```python
from build123d import *

# Parameters (mm, degrees)
BOSS_EXTRUDE1_DEPTH = 20
SKETCH2_R           = 5
BOSS_EXTRUDE2_DEPTH = 10
SKETCH3_R           = 11.25
CUT_EXTRUDE1_DEPTH  = 10
FILLET1_R           = 2.5
FILLET2_R           = 2.5


with BuildPart() as part:
    # Sketch1 → Boss-Extrude1 (new body)
    with BuildSketch(Plane.XY):
        with BuildLine():
            Line((-49.078947743, 24.658688111), (-53.195876289, 25))
            ThreePointArc((-53.195876289, 25), (-78.174127632, -1.04257365), (-51.112542955, -24.913043215))
            Line((-51.112542955, -24.913043215), (68.054123711, -14.947825929))
            ThreePointArc((68.054123711, -14.947825929), (81.804122753, 0.005360617), (68.04343945, 14.948715547))
            Line((68.04343945, 14.948715547), (-49.078947743, 24.658688111))
        make_face()
    extrude(amount=BOSS_EXTRUDE1_DEPTH)

    # Sketch2 → Boss-Extrude2 (add)
    with BuildSketch(Plane(origin=(0, 0, 0), x_dir=(-1, 0, 0), z_dir=(0, 0, -1))):
        with Locations(Location((-66.804123711, 0, 0), (0, 0, 180))):
            Circle(SKETCH2_R)
    extrude(amount=BOSS_EXTRUDE2_DEPTH)

    # Sketch3 → Cut-Extrude1 (cut)
    with BuildSketch(Plane.XY.offset(20)):
        with Locations((-53.195876289, 0)):
            Circle(SKETCH3_R)
    extrude(amount=-CUT_EXTRUDE1_DEPTH, mode=Mode.SUBTRACT)

    # Fillet1
    # the kernel refuses this fillet: 2.5 mm, written as the material it takes off along each edge
    with BuildSketch(Plane(origin=(66.804123711, 0, 20), x_dir=(0.08333333333333336, -0.9965217285917832, 0), z_dir=(-0.9965217285917832, -0.08333333333333336, 0))) as fillet1_piece_1:
        with BuildLine():
            CenterArc((15 - FILLET1_R, -FILLET1_R), FILLET1_R, 0, 90)
            Line((15 - FILLET1_R, 0), (15 - FILLET1_R, FILLET1_R * 0.02))
            Line((15 - FILLET1_R, FILLET1_R * 0.02), (15 + FILLET1_R * 0.02, FILLET1_R * 0.02))
            Line((15 + FILLET1_R * 0.02, FILLET1_R * 0.02), (15 + FILLET1_R * 0.02, -FILLET1_R))
            Line((15 + FILLET1_R * 0.02, -FILLET1_R), (15, -FILLET1_R))
        make_face()
    revolve(axis=Axis((66.804123711, 0, 20), (0, 0, 1)), revolution_arc=170.480568403, mode=Mode.SUBTRACT)
    with BuildSketch(Plane(origin=(-55.68732888, 25.206552623, 20), x_dir=(-0.08262104926117214, -0.9965810364536258, 0), z_dir=(0.9965810364536258, -0.08262104926117214, 0))) as fillet1_piece_2:
        with BuildLine():
            CenterArc((FILLET1_R, FILLET1_R), FILLET1_R, 180, 90)
            Line((0, FILLET1_R), (-FILLET1_R * 0.02, FILLET1_R))
            Line((-FILLET1_R * 0.02, FILLET1_R), (-FILLET1_R * 0.02, -FILLET1_R * 0.02))
            Line((-FILLET1_R * 0.02, -FILLET1_R * 0.02), (FILLET1_R, -FILLET1_R * 0.02))
            Line((FILLET1_R, -FILLET1_R * 0.02), (FILLET1_R, 0))
        make_face()
    extrude(amount=124.155250606, mode=Mode.SUBTRACT)
    with BuildSketch(Plane(origin=(-53.195876289, 0, 20), x_dir=(0.10000205270336067, 0.994987230800031, 0), z_dir=(0.994987230800031, -0.10000205270336067, 0))) as fillet1_piece_3:
        with BuildLine():
            CenterArc((25 - FILLET1_R, -FILLET1_R), FILLET1_R, 0, 90)
            Line((25 - FILLET1_R, 0), (25 - FILLET1_R, FILLET1_R * 0.02))
            Line((25 - FILLET1_R, FILLET1_R * 0.02), (25 + FILLET1_R * 0.02, FILLET1_R * 0.02))
            Line((25 + FILLET1_R * 0.02, FILLET1_R * 0.02), (25 + FILLET1_R * 0.02, -FILLET1_R))
            Line((25 + FILLET1_R * 0.02, -FILLET1_R), (25, -FILLET1_R))
        make_face()
    revolve(axis=Axis((-53.195876289, 0, 20), (0, 0, 1)), revolution_arc=190.519480528, mode=Mode.SUBTRACT)
    with BuildSketch(Plane(origin=(-51.112542955, -24.913043215, 20), x_dir=(0, 0, -1), z_dir=(0.9965217285917832, 0.08333333333333336, 0))) as fillet1_piece_4:
        with BuildLine():
            CenterArc((FILLET1_R, FILLET1_R), FILLET1_R, 180, 90)
            Line((0, FILLET1_R), (-FILLET1_R * 0.02, FILLET1_R))
            Line((-FILLET1_R * 0.02, FILLET1_R), (-FILLET1_R * 0.02, -FILLET1_R * 0.02))
            Line((-FILLET1_R * 0.02, -FILLET1_R * 0.02), (FILLET1_R, -FILLET1_R * 0.02))
            Line((FILLET1_R, -FILLET1_R * 0.02), (FILLET1_R, 0))
        make_face()
    extrude(amount=119.582607431, mode=Mode.SUBTRACT)

    # Fillet2
    # the kernel refuses this fillet: 2.5 mm, written as the material it takes off along each edge
    with BuildSketch(Plane(origin=(-53.195876289, 0, 0), x_dir=(0.10000205270336067, 0.994987230800031, 0), z_dir=(0.994987230800031, -0.10000205270336067, 0))) as fillet2_piece_1:
        with BuildLine():
            CenterArc((25 - FILLET2_R, FILLET2_R), FILLET2_R, 270, 90)
            Line((25, FILLET2_R), (25 + FILLET2_R * 0.02, FILLET2_R))
            Line((25 + FILLET2_R * 0.02, FILLET2_R), (25 + FILLET2_R * 0.02, -FILLET2_R * 0.02))
            Line((25 + FILLET2_R * 0.02, -FILLET2_R * 0.02), (25 - FILLET2_R, -FILLET2_R * 0.02))
            Line((25 - FILLET2_R, -FILLET2_R * 0.02), (25 - FILLET2_R, 0))
        make_face()
    revolve(axis=Axis((-53.195876289, 0, 0), (0, 0, 1)), revolution_arc=190.519480528, mode=Mode.SUBTRACT)
    with BuildSketch(Plane(origin=(68.04343945, 14.948715547, 0), x_dir=(-0.08262104926117214, -0.9965810364536258, 0), z_dir=(-0.9965810364536258, 0.08262104926117214, 0))) as fillet2_piece_2:
        with BuildLine():
            CenterArc((FILLET2_R, FILLET2_R), FILLET2_R, 180, 90)
            Line((0, FILLET2_R), (-FILLET2_R * 0.02, FILLET2_R))
            Line((-FILLET2_R * 0.02, FILLET2_R), (-FILLET2_R * 0.02, -FILLET2_R * 0.02))
            Line((-FILLET2_R * 0.02, -FILLET2_R * 0.02), (FILLET2_R, -FILLET2_R * 0.02))
            Line((FILLET2_R, -FILLET2_R * 0.02), (FILLET2_R, 0))
        make_face()
    extrude(amount=124.155250606, mode=Mode.SUBTRACT)
    with BuildSketch(Plane(origin=(66.804123711, 0, 0), x_dir=(0.08333333333333336, -0.9965217285917832, 0), z_dir=(-0.9965217285917832, -0.08333333333333336, 0))) as fillet2_piece_3:
        with BuildLine():
            CenterArc((15 - FILLET2_R, FILLET2_R), FILLET2_R, 270, 90)
            Line((15, FILLET2_R), (15 + FILLET2_R * 0.02, FILLET2_R))
            Line((15 + FILLET2_R * 0.02, FILLET2_R), (15 + FILLET2_R * 0.02, -FILLET2_R * 0.02))
            Line((15 + FILLET2_R * 0.02, -FILLET2_R * 0.02), (15 - FILLET2_R, -FILLET2_R * 0.02))
            Line((15 - FILLET2_R, -FILLET2_R * 0.02), (15 - FILLET2_R, 0))
        make_face()
    revolve(axis=Axis((66.804123711, 0, 0), (0, 0, 1)), revolution_arc=170.480568403, mode=Mode.SUBTRACT)
    with BuildSketch(Plane(origin=(-51.112542955, -24.913043215, 0), x_dir=(0, 0, 1), z_dir=(0.9965217285917832, 0.08333333333333336, 0))) as fillet2_piece_4:
        with BuildLine():
            CenterArc((FILLET2_R, -FILLET2_R), FILLET2_R, 90, 90)
            Line((0, -FILLET2_R), (-FILLET2_R * 0.02, -FILLET2_R))
            Line((-FILLET2_R * 0.02, -FILLET2_R), (-FILLET2_R * 0.02, FILLET2_R * 0.02))
            Line((-FILLET2_R * 0.02, FILLET2_R * 0.02), (FILLET2_R, FILLET2_R * 0.02))
            Line((FILLET2_R, FILLET2_R * 0.02), (FILLET2_R, 0))
        make_face()
    extrude(amount=119.582607431, mode=Mode.SUBTRACT)


solid = part.part
```
Source: CAD feature listing. Evaluate the final solid. Frame: model axes, mm. A direction names the side the tool comes from. Give positions to 0.01 mm unless a question says otherwise; leave off trailing zeros. Loops run counter-clockwise (first coordinate to the right, second up) from the corner with the lowest first, then second, coordinate; pieces in that order, holes last. Notation, with made-up numbers: (48.25, -28) -> (99.25, -28) arc R14 ccw to (99.25, -17) -> close; hole circle Ø10 at (8, 68.5). An arc over 180 degrees is marked (long way). Use a Markdown table: item, result. Add a question column.
(1) Section query B-B (y = 0). Output: boundary loops of the cut face in (x, z).
(2) Pull-direction query (X, two-part tool) for faces 1 (the face through (-53, 0, 10)), 2 (the face through (7.57, -19.25, 19.29)), 3 (the face through (1, 0, 0)); classes: +X half, -X half, draft (parallel to the pull), parting line (faces both ways), or undercut.
(3) Section query A-A (z = 12). Output: boundary loops of the cut face in (x, y).
(4) Ray query, line 1 (Y direction, x = -48.5, z = 16); line 2 (Z direction, x = 24, y = -6); line 3 (Y direction, x = -50.5, z = 15). Return the intervals inside material, ascending.
(5) First-contact query: pin 1 Ø11 at (x, y) = (-54, 1.5) entering from +Z; pin 2 Ø3 at (x, y) = (33.5, -9) entering from -Z; pin 3 Ø2 at (y, z) = (9.5, 1) entering from +X; pin 4 Ø3 at (x, y) = (-0.5, 19) entering from +Z. Flat tips, straight axial feed; report the tip coordinate or a pass-through.
(6) Access query for faces 4 (the face through (61.81, -0.22, -4.93)), 5 (the face through (1, 0, 20)), 6 (the face through (-62.12, -6.85, 15.07)). Directions: +Z, -Z, +X, -X, +Y, -Y. A direction counts if a zero-diameter tool reaches every point of the face in a straight line with its end or side. Return the directions, or none.
(7) Section query C-C (z = -1.5). Output: boundary loops of the cut face in (x, y), then the cut area to 3 significant figures.
Checked values:
| question | item | result |
|---|---|---|
| 1 | outline | (-78.2, 2.5) arc R2.5 ccw to (-75.7, 0) -> (61.8, 0) -> (61.8, -10) -> (71.8, -10) -> (71.8, 0) -> (79.3, 0) arc R2.5 ccw to (81.8, 2.5) -> (81.8, 17.5) arc R2.5 ccw to (79.3, 20) -> (-41.95, 20) -> (-41.95, 10) -> (-64.45, 10) -> (-64.45, 20) -> (-75.7, 20) arc R2.5 ccw to (-78.2, 17.5) -> close |
| 2 | face 1 | undercut |
| 2 | face 2 | +X half |
| 2 | face 3 | draft |
| 3 | outline | (-53.2, 25) arc R25 ccw (long way) to (-51.11, -24.91) -> (68.05, -14.95) arc R15 ccw to (68.04, 14.95) -> close; hole circle Ø22.5 at (-53.2, 0) |
| 4 | line 1 | -24.69 to -10.22, 10.22 to 24.61 |
| 4 | line 2 | 0 to 20 |
| 4 | line 3 | -24.86 to -10.92, 10.92 to 24.78 |
| 5 | pin 1 | z = 10 |
| 5 | pin 2 | z = 0 |
| 5 | pin 3 | x = 78.82 |
| 5 | pin 4 | z = 20 |
| 6 | face 4 | -Z |
| 6 | face 5 | +Z, +X, -X, +Y, -Y |
| 6 | face 6 | +Z |
| 7 | outline | circle Ø10 at (66.8, 0) |
| 7 | area | 78.5 mm^2 |
